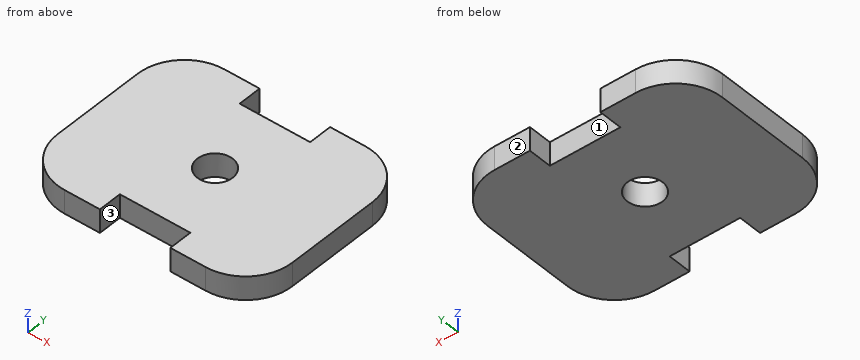
from build123d import *

# Parameters (mm, degrees)
SKETCH1_R           = 2.38125
BOSS_EXTRUDE1_DEPTH = 3.175


with BuildPart() as part:
    # Sketch1 → Boss-Extrude1 (new body)
    with BuildSketch(Plane.XY):
        with BuildLine():
            Line((1.5875, 21.137006158), (-3.175, 21.137006158))
            ThreePointArc((-3.175, 21.137006158), (-7.665128061, 19.277134219), (-9.525, 14.787006158))
            Line((-9.525, 14.787006158), (-9.525, 2.087006158))
            ThreePointArc((-9.525, 2.087006158), (-7.665128061, -2.403121902), (-3.175, -4.262993842))
            Line((-3.175, -4.262993842), (1.5875, -4.262993842))
            Line((1.5875, -4.262993842), (1.5875, -1.087993842))
            Line((1.5875, -1.087993842), (11.1125, -1.087993842))
            Line((11.1125, -1.087993842), (11.1125, -4.262993842))
            Line((11.1125, -4.262993842), (15.875, -4.262993842))
            ThreePointArc((15.875, -4.262993842), (20.365128061, -2.403121902), (22.225, 2.087006158))
            Line((22.225, 2.087006158), (22.225, 14.787006158))
            ThreePointArc((22.225, 14.787006158), (20.365128061, 19.277134219), (15.875, 21.137006158))
            Line((15.875, 21.137006158), (11.1125, 21.137006158))
            Line((11.1125, 21.137006158), (11.1125, 17.962006158))
            Line((11.1125, 17.962006158), (1.5875, 17.962006158))
            Line((1.5875, 17.962006158), (1.5875, 21.137006158))
        make_face()
        with Locations((6.35, 8.437006158)):
            Circle(SKETCH1_R, mode=Mode.SUBTRACT)
    extrude(amount=BOSS_EXTRUDE1_DEPTH)


solid = part.part
Could you check a few things on this model? Use its own coordinates, in mm. Face numbers are marked on the shaded views. A direction names the side the tool comes from. Give positions to 0.01 mm unless a question says otherwise; leave off trailing zeros. Order: outer loops, then holes, each group sorted by start corner. A loop starts at its lowest first (then second) coordinate and runs counter-clockwise, first axis right, second up. Notation, with made-up numbers: (-20, -34) -> (27, -34) arc R18 cw to (27, -26) -> close; hole circle Ø4 at (31.25, 27). An arc over 180 degrees is marked (long way). Return JSON: item names as keys, results as strings.
1. On a 3-axis mill with a long thin cutter (end or side, diameter ignored), from which of +Z, -Z, +X, -X, +Y, -Y can I reach the whole of each face in a straight line? I mean the marked faces 1, 2 and 3. Say none if no direction works.
Answer list:
{"face 1": "+Z, -Z, +Y", "face 2": "+Z, -Z, +X, -X, +Y", "face 3": "+Z, -Z, -Y"}
2. Imagine slicing it at B-B on y = 6.5. List the corners of the cut face in (x, z) for me (3 decimals), then the cut area to 3 significant figures.
Answer list:
{"outline": "(-9.525, 0) -> (4.965, 0) -> (4.965, 3.175) -> (-9.525, 3.175) -> close; (7.735, 0) -> (22.225, 0) -> (22.225, 3.175) -> (7.735, 3.175) -> close", "area": "92.0 mm2"}
3. I need wall thicknesses on line 1 (Y direction, x = 6.35, z = 2.2); line 2 (X direction, y = 19.5, z = 2.95); line 3 (X direction, y = 9, z = 1.9) (3 decimals). Which ranges of each line are inside material? Lowest first, please. Write a range as from..to.
Answer list:
{"line 1": "y = -1.09..6.06, 10.82..17.96", "line 2": "x = -7.43..1.59, 11.11..20.13", "line 3": "x = -9.525..4.036, 8.664..22.225"}
4. Imagine slicing it at D-D on x = -6. List the corners of the cut face in (y, z) for me (3 decimals).
Answer list:
{"outline": "(-3.6, 0) -> (20.474, 0) -> (20.474, 3.175) -> (-3.6, 3.175) -> close"}
5. Imagine slicing it at A-A on x = 6.35. List the corners of the cut face in (y, z) for me (3 decimals).
Answer list:
{"outline": "(-1.088, 0) -> (6.056, 0) -> (6.056, 3.175) -> (-1.088, 3.175) -> close; (10.818, 0) -> (17.962, 0) -> (17.962, 3.175) -> (10.818, 3.175) -> close"}
6. For pin 1 Ø1 at (y, z) = (-2, 1.5) entering from -X; pin 2 Ø7.5 at (x, y) = (6.35, 8.44) entering from -Z; pin 3 Ø1.6 at (y, z) = (-2, 1.5) entering from +X; pin 4 Ø1.6 at (x, z) = (6.5, 1) entering from +Y, each with a flat end and sliding along its axis, tell me the tip position at first contact or that it passes through.
Answer list:
{"pin 1": "stops at x = -8.41", "pin 2": "stops at z = 0", "pin 3": "stops at x = 21.31", "pin 4": "stops at y = 17.96"}
